Answer from the drawing. Dimensions are ordinates in mm from the lowest x, y and z of the part. Round coordinates to 2 decimals unless told otherwise and drop trailing zeros. Loops run counter-clockwise (first coordinate to the right, second up) from the corner with the lowest first, then second, coordinate; pieces in that order, holes last. Notation, with made-up numbers: (13.5, -35) - (23.5, -35) arc R12 ccw to (23.5, -18) - close; hole circle Ø11 at (-34.75, 52). An arc over 180 degrees is marked (long way). Return JSON: item names as keys, results as strings.
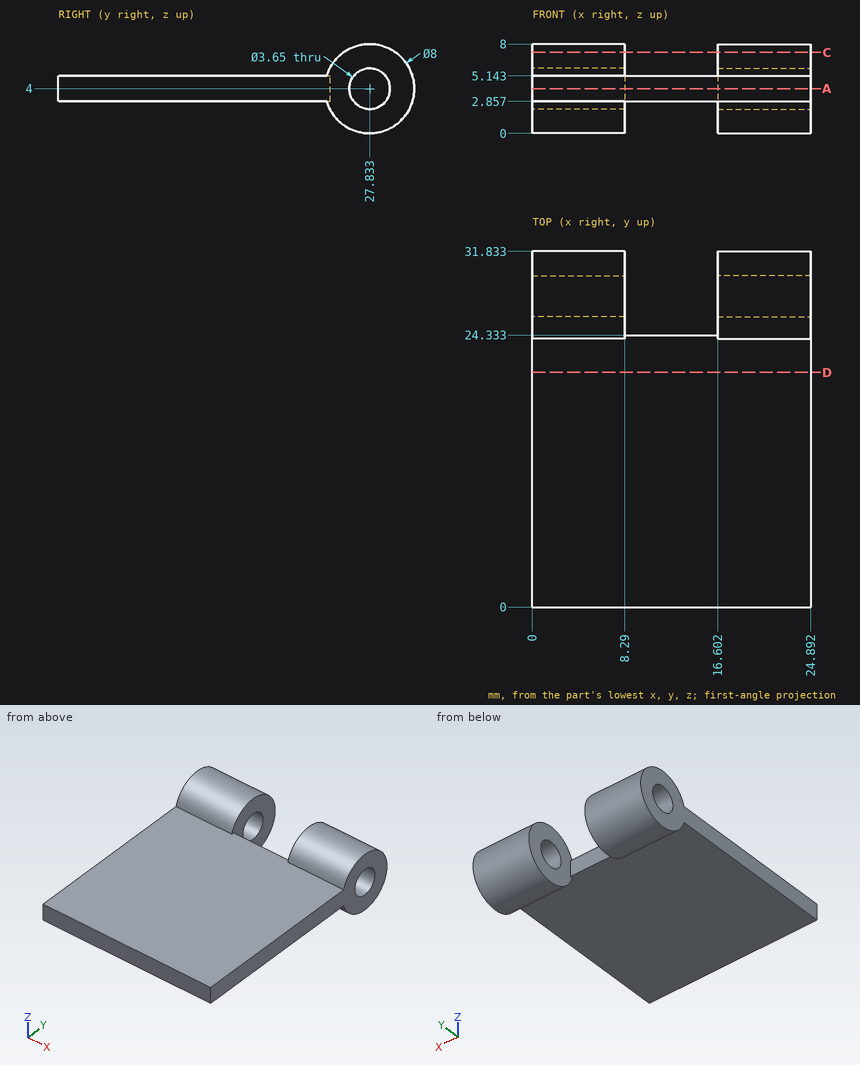
1) Section C-C (z = 7.25) is taken. Give the vertices of the cut face in (x, y) (1 decimal).
Verdict:
{"outline": "(0, 25.5) - (8.3, 25.5) - (8.3, 30.2) - (0, 30.2) - close; (16.6, 25.5) - (24.9, 25.5) - (24.9, 30.2) - (16.6, 30.2) - close"}
2) Flat-ended cylindrical pins translate along their axes: pin 1 (12 mm diameter, centred on x = 12.5, y = 11, fed in from -Z); pin 2 (5 mm diameter, centred on x = 21, y = 9, fed in from +Z); pin 3 (2.5 mm diameter, centred on x = 11.5, z = 4.5, fed in from +Y). Find the tip coordinate at first contact, or state that the pin passes through.
Verdict:
{"pin 1": "stops at z = 2.86", "pin 2": "stops at z = 5.14", "pin 3": "stops at y = 24.33"}
3) Find the intervals of material crossed by L1, parallel to Z at x = 23, y = 9; L2, parallel to Y at x = 18.75, z = 5.25; L3, parallel to Y at x = 22.25, z = 3, in increasing order.
Verdict:
{"L1": "z = 2.86 to 5.14", "L2": "y = 24.03 to 26.5, 29.16 to 31.63", "L3": "y = 0 to 26.31, 29.36 to 31.71"}
4) Section D-D (y = 21) is taken. Give the vertices of the cut face in (x, z), and give its area (3 significant figures).
Verdict:
{"outline": "(0, 2.86) - (24.89, 2.86) - (24.89, 5.14) - (0, 5.14) - close", "area": "56.9 mm2"}
5) Section A-A (z = 4) is taken. Give the vertices of the cut face in (x, y).
Verdict:
{"outline": "(0, 0) - (24.89, 0) - (24.89, 26.01) - (16.6, 26.01) - (16.6, 24.33) - (8.29, 24.33) - (8.29, 26.01) - (0, 26.01) - close; (0, 29.66) - (8.29, 29.66) - (8.29, 31.83) - (0, 31.83) - close; (16.6, 29.66) - (24.89, 29.66) - (24.89, 31.83) - (16.6, 31.83) - close"}
